Can you work these out from the drawing? Everything is in mm from the part's minimum corner. A direction names the side the tool comes from. Round coordinates to 2 decimals unless told otherwise and drop trailing zeros. Write each loop counter-clockwise with the first axis right and the second up, starting at its lowest first coordinate (ties: lowest second). Pieces come first, ordered by that corner, then holes.
Q1. If we section it at B-B (x = 2.5): Please give me the cut outline in (y, z), plus the area to 4 significant figures.
Q2. Please list where these lines run through material, in increasing order: line 1 along Z through (x, y) = (1.75, 2.2); line 2 along Y through (x, z) = (7.25, 1.3); line 3 along X through (y, z) = (2.4, 0.85).
Q3. If we section it at C-C (z = 0.4): Please give me the cut outline in (x, y), plus the area to 3 significant figures.
Q4. For the marked faces 1, 2, 3 and 4, which set-ups out of +Z, -Z, +X, -X, +Y, -Y let a thin tool reach every point of the face, with its end or its side?
Q5. I'm going to push flat-ended pins straight in: pin 1 Ø1.5 at (x, y) = (4.5, 0.5) entering from +Z; pin 2 Ø1.5 at (x, y) = (1.5, 0.5) entering from -Z; pin 3 Ø1.8 at (x, z) = (2.5, 1.5) entering from -Y; pin 4 Ø1 at (y, z) = (1.5, 2) entering from +X. Where does each tip first touch, or does it pass through?
Q6. We'd pull the mould along Z, two halves only. Please class the marked faces 5, 6 and 7: +Z half, -Z half, draft (parallel to the pull), parting line (faces both ways), or undercut.
Q7. If we section it at A-A (z = 2.2): Please give me the cut outline in (x, y), plus the area to 3 significant figures.
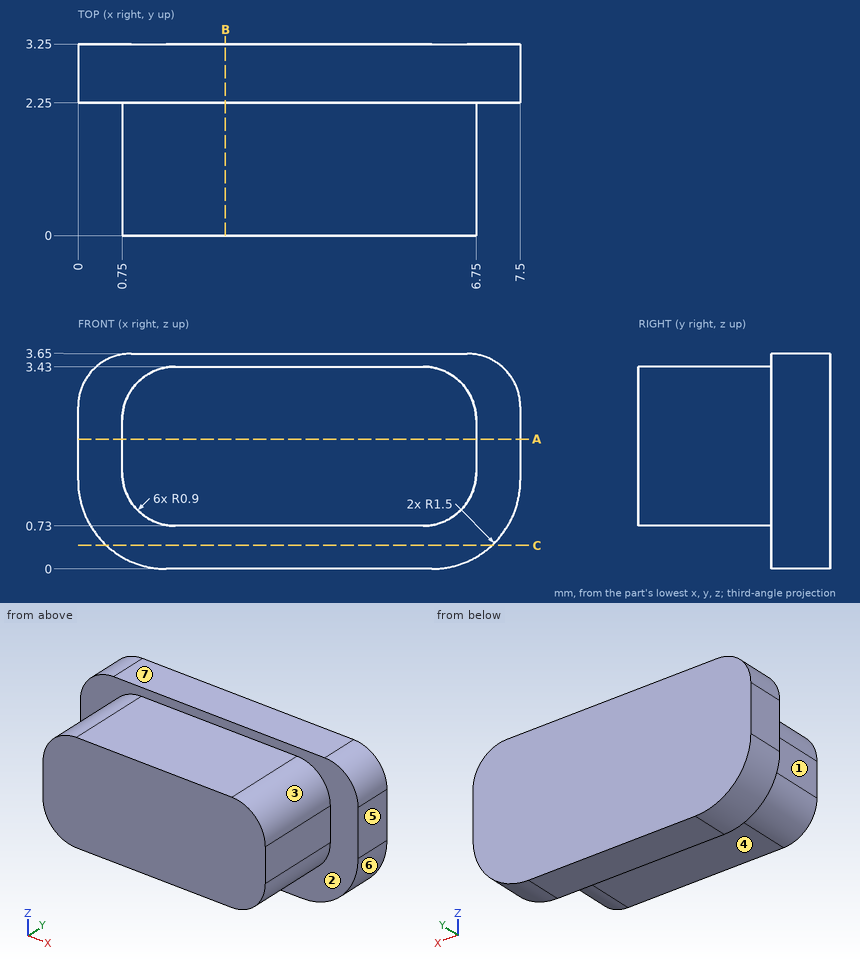
A:
1. outline: (0, 0.73) - (2.25, 0.73) - (2.25, 0) - (3.25, 0) - (3.25, 3.65) - (2.25, 3.65) - (2.25, 3.43) - (0, 3.43) - close
1. area: 9.725 mm2
2. line 1: z = 0.73 to 3.43
2. line 2: y = 2.25 to 3.25
2. line 3: x = 0.15 to 7.35
3. outline: (0.48, 2.25) - (7.02, 2.25) - (7.02, 3.25) - (0.48, 3.25) - close
3. area: 6.54 mm2
4. face 1: +Z, -Z, -X, -Y
4. face 2: -Y
4. face 3: +Z, +X, -Y
4. face 4: -Z, +X, -X, -Y
5. pin 1: stops at z = 3.43
5. pin 2: stops at z = 0.73
5. pin 3: stops at y = 0
5. pin 4: stops at x = 6.75
6. face 5: draft
6. face 6: -Z half
6. face 7: +Z half
7. outline: (0, 2.25) - (0.75, 2.25) - (0.75, 0) - (6.75, 0) - (6.75, 2.25) - (7.5, 2.25) - (7.5, 3.25) - (0, 3.25) - close
7. area: 21.0 mm2
